Build history of the part. All positions in model axes, mm. A direction names the side the tool comes from. Give positions to 0.01 mm unless a question says otherwise; leave off trailing zeros. Loops run counter-clockwise (first coordinate to the right, second up) from the corner with the lowest first, then second, coordinate; pieces in that order, holes last. Notation, with made-up numbers: (17.25, 11.5) -> (40.25, 11.5) arc R25 cw to (40.25, 43.5) -> close; hole circle Ø11 at (85.25, -3.5). An arc over 180 degrees is marked (long way). One line per question, with ' | ' between items. Start each with the question number.
(1) Drill centre lines: L1, parallel to X at y = -5, z = 2.5; L2, parallel to Y at x = -34, z = 1; L3, parallel to Z at x = -31.5, y = 5 (3 decimals). Where is each one in solid material? Low to high. Write a range as from..to.
(2) Slice it at B-B, the plane z = 5.75. Write the cut outline in (x, y), then the cut area to 3 significant figures.
(3) Slice it at D-D, the plane y = 12. Write the cut outline in (x, z) (1 decimal).
(4) Slice it at C-C, the plane x = -11. Write the cut outline in (y, z) (1 decimal), then the cut area to 3 significant figures.
(5) 3-axis set-ups, long thin cutter, end or side, ignore diameter. For faces 1 (the face through (-21.9, 51.7, 1.588)), 2 (the face through (-33, 37.505, 2)), 3 (the face through (-14.31, 14.69, 4.94)): which of +Z, -Z, +X, -X, +Y, -Y reach the whole face in a straight line?
(6) Slice it at A-A, the plane x = 4.5. Write the cut outline in (y, z) (1 decimal), then the cut area to 3 significant figures.
(7) Flat gauge pins, fed straight in: pin 1 Ø6 at (x, y) = (-23.5, 43.5) entering from -Z; pin 2 Ø1.7 at (y, z) = (39, 2.5) entering from -X; pin 3 Ø1.7 at (x, z) = (-8, 2.5) entering from -Y; pin 4 Ø3.5 at (x, y) = (-21.5, 51) entering from +Z. Where does each tip first touch, or does it go through?
(8) Mould opens along X. For faces 4 (the face through (-22.97, 21.01, 4.94)), 5 (the face through (-14.46, 29.388, 3.421)), 6 (the face through (-7, -1.588, 2)), 7 (the face through (5.674, -5.551, 1.565)) say: pulls with the +X half, pulls with the -X half, needs draft (parallel to the pull), parting line crosses it, or undercut.
Autodesk Inventor part; units mm, degrees
ref_plane "YZ Plane" through (0, 0, 0) normal (1, 0, 0) x (0, 1, 0)
ref_plane "XZ Plane" through (0, 0, 0) normal (0, 1, 0) x (-1, 0, 0)
ref_plane "XY Plane" through (0, 0, 0) normal (0, 0, 1) x (1, 0, 0)
sketch "Sketch27" plane through (0, 0, 0) normal (0, 0, 1) x (1, 0, 0)
  line L0 (0, -7.9375) -> (-28.575, -7.9375)
  line L1 (-36.5125, 0) -> (-36.5125, 47.625)
  line L2 (-28.575, 55.5625) -> (0, 55.5625)
  line L3 (7.9375, 47.625) -> (7.9375, 0)
  circle A0 centre (-28.575, 47.625) radius 6.5484
  circle A1 centre (-28.575, 31.75) radius 6.5484
  circle A2 centre (-28.575, 15.875) radius 6.5484
  circle A3 centre (-28.575, 0) radius 6.5484
  circle A4 centre (-14.2875, 0) radius 6.5484
  circle A5 centre (-14.2875, 47.625) radius 6.5484
  circle A6 centre (0, 47.625) radius 6.5484
  circle A7 centre (0, 31.75) radius 6.5484
  circle A8 centre (0, 15.875) radius 6.5484
  circle A9 centre (0, 0) radius 6.5484
  arc A10 (-28.575, 55.5625) -> (-36.5125, 47.625) centre (-28.575, 47.625) ccw
  arc A11 (7.9375, 47.625) -> (0, 55.5625) centre (0, 47.625) ccw
  arc A12 (-36.5125, 0) -> (-28.575, -7.9375) centre (-28.575, 0) ccw
  arc A13 (0, -7.9375) -> (7.9375, 0) centre (0, 0) ccw
  circle A14 centre (-33.3375, 39.6875) radius 1.3891
  circle A15 centre (-33.3375, 23.8125) radius 1.3891
  circle A16 centre (-33.3375, 7.9375) radius 1.3891
  circle A17 centre (4.7625, 39.6875) radius 1.3891
  circle A18 centre (4.7625, 23.8125) radius 1.3891
  circle A19 centre (4.7625, 7.9375) radius 1.3891
  circle A20 centre (-21.4312, 53.1812) radius 1.3891
  circle A21 centre (-7.1437, 53.1812) radius 1.3891
  circle A22 centre (-21.4312, -5.5562) radius 1.3891
  circle A23 centre (-7.1437, -5.5562) radius 1.3891
  dimension "d126" = 13.0969
  dimension "d127" = 13.0969
  dimension "d128" = 13.0969
  dimension "d129" = 13.0969
  dimension "d130" = 13.0969
  dimension "d131" = 13.0969
  dimension "d132" = 13.0969
  dimension "d133" = 13.0969
  dimension "d134" = 13.0969
  dimension "d135" = 13.0969
  dimension "d136" = 7.9375
  dimension "d137" = 14.2875
  dimension "d138" = 14.2875
  dimension "d139" = 7.9375
  dimension "d140" = 7.9375
  dimension "d141" = 15.875
  dimension "d142" = 15.875
  dimension "d145" = 44.45
  dimension "d146" = 63.5
  dimension "d149" = 2.7781
  dimension "d150" = 2.7781
  dimension "d151" = 2.7781
  dimension "d152" = 2.7781
  dimension "d153" = 2.7781
  dimension "d154" = 2.7781
  dimension "d155" = 3.175
  dimension "d156" = 3.175
  dimension "d157" = 15.875
  dimension "d158" = 15.875
  dimension "d159" = 15.875
  dimension "d162" = 2.7781
  dimension "d163" = 2.7781
  dimension "d164" = 2.7781
  dimension "d165" = 2.7781
  dimension "d166" = 2.3813
  dimension "d169" = 2.3813
  dimension "d170" = 7.1437
  dimension "d171" = 7.1437
extrude "Extrusion25" add sketch "Sketch27" along normal blind 3.175 contours L0 A12 L1 A10 L2 A11 L3 A13 | A0 | A1 | A2 | A3 | A4 | A5 | A6 | A7 | A8 | A9
sketch "Sketch38" plane through (0, 0, 3.175) normal (0, 0, 1) x (1, 0, 0)
  circle A0 centre (-14.2875, 23.8125) radius 9.525
  arc A1 (-15.4885, 33.2615) -> (-18.8698, 32.1628) centre (-16.6896, 31.2053) ccw
  arc A2 (-15.4885, 33.2615) -> (-13.0865, 33.2615) centre (-14.2875, 35.3177) ccw
  line L0 (7.9375, 0) -> (7.9375, 47.625)
  line L1 (0, 55.5625) -> (-28.575, 55.5625)
  arc A3 (-9.7052, 32.1628) -> (-13.0865, 33.2615) centre (-11.8854, 31.2053) ccw
  arc A4 (-9.7052, 32.1628) -> (-7.7619, 30.7509) centre (-7.5249, 33.1204) ccw
  arc A5 (-5.6721, 27.8746) -> (-7.7619, 30.7509) centre (-7.9988, 28.3815) ccw
  arc A6 (-5.6721, 27.8746) -> (-4.9299, 25.5901) centre (-3.3454, 27.3678) ccw
  arc A7 (-4.9299, 22.0349) -> (-4.9299, 25.5901) centre (-6.5143, 23.8125) ccw
  arc A8 (-4.9299, 22.0349) -> (-5.6721, 19.7504) centre (-3.3454, 20.2572) ccw
  arc A9 (-7.7619, 16.8741) -> (-5.6721, 19.7504) centre (-7.9988, 19.2435) ccw
  arc A10 (-7.7619, 16.8741) -> (-9.7052, 15.4622) centre (-7.5249, 14.5046) ccw
  arc A11 (-13.0865, 14.3635) -> (-9.7052, 15.4622) centre (-11.8854, 16.4197) ccw
  arc A12 (-13.0865, 14.3635) -> (-15.4885, 14.3635) centre (-14.2875, 12.3073) ccw
  arc A13 (-18.8698, 15.4622) -> (-15.4885, 14.3635) centre (-16.6896, 16.4197) ccw
  arc A14 (-18.8698, 15.4622) -> (-20.8131, 16.8741) centre (-21.0501, 14.5046) ccw
  arc A15 (-22.9029, 19.7504) -> (-20.8131, 16.8741) centre (-20.5762, 19.2435) ccw
  arc A16 (-22.9029, 19.7504) -> (-23.6451, 22.0349) centre (-25.2296, 20.2572) ccw
  arc A17 (-20.8131, 30.7509) -> (-18.8698, 32.1628) centre (-21.0501, 33.1204) ccw
  arc A18 (-23.6451, 25.5901) -> (-23.6451, 22.0349) centre (-22.0607, 23.8125) ccw
  arc A19 (-23.6451, 25.5901) -> (-22.9029, 27.8746) centre (-25.2296, 27.3678) ccw
  arc A20 (-20.8131, 30.7509) -> (-22.9029, 27.8746) centre (-20.5762, 28.3815) ccw
  point P0 (0, 0)
  dimension "d265" = 19.05
  dimension "d266" = 22.225
  dimension "d267" = 31.75
  dimension "d268" = 2.3813
extrude "Extrusion29" add sketch "Sketch38" along normal blind 3.5719 contours A0 A8 A10 A12 A14 A16 A19 A17 A2 A4 A6 | A0 A7 | A0 A5 | A9 A0 | A0 A3 | A11 A0 | A0 A1 | A13 A0 | A0 A20 | A15 A0 | A0 A18
sketch "Sketch39" plane through (0, 0, 3.175) normal (0, 0, 1) x (1, 0, 0)
  line L0 (7.9375, 10.1203) -> (1.5875, 10.1203)
  line L1 (1.5875, 10.1203) -> (1.5875, 5.7547)
  line L2 (1.5875, 5.7547) -> (7.9375, 5.7547)
  line L3 (7.9375, 5.7547) -> (7.9375, 10.1203)
  line L4 (7.9375, 0) -> (7.9375, 47.625)
  circle A0 centre (4.7625, 7.9375) radius 1.3891
  line L5 (7.9375, 25.9953) -> (1.5875, 25.9953)
  line L6 (1.5875, 25.9953) -> (1.5875, 21.6297)
  line L7 (1.5875, 21.6297) -> (7.9375, 21.6297)
  line L8 (7.9375, 21.6297) -> (7.9375, 25.9953)
  line L9 (7.9375, 41.8703) -> (1.5875, 41.8703)
  line L10 (1.5875, 41.8703) -> (1.5875, 37.5047)
  line L11 (1.5875, 37.5047) -> (7.9375, 37.5047)
  line L12 (7.9375, 37.5047) -> (7.9375, 41.8703)
  line L13 (0, 55.5625) -> (-28.575, 55.5625)
  line L14 (-9.3266, 55.5625) -> (-4.9609, 55.5625)
  line L15 (-4.9609, 55.5625) -> (-4.9609, 49.2125)
  line L16 (-4.9609, 49.2125) -> (-9.3266, 49.2125)
  line L17 (-9.3266, 49.2125) -> (-9.3266, 55.5625)
  line L18 (-19.2484, 55.5625) -> (-23.6141, 55.5625)
  line L19 (-23.6141, 55.5625) -> (-23.6141, 49.2125)
  line L20 (-23.6141, 49.2125) -> (-19.2484, 49.2125)
  line L21 (-19.2484, 49.2125) -> (-19.2484, 55.5625)
  line L22 (-36.5125, 41.8703) -> (-30.1625, 41.8703)
  line L23 (-30.1625, 41.8703) -> (-30.1625, 37.5047)
  line L24 (-30.1625, 37.5047) -> (-36.5125, 37.5047)
  line L25 (-36.5125, 37.5047) -> (-36.5125, 41.8703)
  line L26 (-36.5125, 25.9953) -> (-30.1625, 25.9953)
  line L27 (-30.1625, 25.9953) -> (-30.1625, 21.6297)
  line L28 (-30.1625, 21.6297) -> (-36.5125, 21.6297)
  line L29 (-36.5125, 21.6297) -> (-36.5125, 25.9953)
  line L30 (-36.5125, 10.1203) -> (-30.1625, 10.1203)
  line L31 (-30.1625, 10.1203) -> (-30.1625, 5.7547)
  line L32 (-30.1625, 5.7547) -> (-36.5125, 5.7547)
  line L33 (-36.5125, 5.7547) -> (-36.5125, 10.1203)
  line L34 (0, -7.9375) -> (-28.575, -7.9375)
  line L35 (-23.6141, -7.9375) -> (-19.2484, -7.9375)
  line L36 (-19.2484, -7.9375) -> (-19.2484, -1.5875)
  line L37 (-19.2484, -1.5875) -> (-23.6141, -1.5875)
  line L38 (-23.6141, -1.5875) -> (-23.6141, -7.9375)
  line L39 (-9.3266, -7.9375) -> (-4.9609, -7.9375)
  line L40 (-4.9609, -7.9375) -> (-4.9609, -1.5875)
  line L41 (-4.9609, -1.5875) -> (-9.3266, -1.5875)
  line L42 (-9.3266, -1.5875) -> (-9.3266, -7.9375)
  line L43 (-36.5125, 47.625) -> (-36.5125, 0)
  circle A1 centre (4.7625, 23.8125) radius 1.3891
  circle A2 centre (4.7625, 39.6875) radius 1.3891
  circle A3 centre (-7.1437, 53.1812) radius 1.3891
  circle A4 centre (-21.4312, 53.1812) radius 1.3891
  point P0 (0, 0)
  dimension "d273" = 4.3656
  dimension "d274" = 6.35
  dimension "d275" = 2.1828
  dimension "d276" = 2.1828
  dimension "d277" = 2.1828
  dimension "d278" = 2.1828
  dimension "d279" = 2.1828
extrude "Extrusion30" cut sketch "Sketch39" against normal blind 1.5875
sketch "Sketch41" plane through (0, 0, 6.7469) normal (0, 0, 1) x (1, 0, 0)
  circle A0 centre (-14.2875, 30.1625) radius 0.7937
  circle A1 centre (-14.2875, 17.4625) radius 0.7937
  circle A2 centre (-7.9375, 23.8125) radius 0.7937
  circle A3 centre (-20.6375, 23.8125) radius 0.7937
  line L0 (-9.3266, 55.5625) -> (-19.2484, 55.5625)
  line L1 (7.9375, 25.9953) -> (7.9375, 37.5047)
  point P0 (0, 0)
  dimension "d287" = 1.5875
  dimension "d288" = 1.5875
  dimension "d289" = 1.5875
  dimension "d290" = 1.5875
  dimension "d291" = 12.7
  dimension "d292" = 12.7
  dimension "d293" = 6.35
  dimension "d294" = 6.35
  dimension "d295" = 25.4
  dimension "d296" = 15.875
extrude "Extrusion32" cut sketch "Sketch41" against normal through all
equation "\"d127\" = d126"
equation "\"d128\" = d126"
equation "\"d129\" = d126"
equation "\"d130\" = d126"
equation "\"d131\" = d126"
equation "\"d132\" = d126"
equation "\"d133\" = d126"
equation "\"d134\" = d126"
equation "\"d135\" = d126"
equation "\"d138\" = d137"
equation "\"d139\" = d136"
equation "\"d140\" = d136"
equation "\"d142\" = d141"
equation "\"d150\" = d149"
equation "\"d151\" = d149"
equation "\"d152\" = d149"
equation "\"d153\" = d149"
equation "\"d154\" = d149"
equation "\"d158\" = d157"
equation "\"d159\" = d157"
equation "\"d162\" = d149"
equation "\"d163\" = d149"
equation "\"d164\" = d149"
equation "\"d165\" = d149"
equation "\"d170\" = 0.5 * d137"
equation "\"d171\" = d170"
properties part number "magnetic1-1"
Final values:
1) L1: -34.74..-23.61, -19.25..-9.33, -4.96..6.16 | L2: -5.79..6.72, 9.16..22.59, 25.03..38.47, 40.91..53.42 | L3: 0..3.175
2) outline: (-23.65, 22.03) arc R2.38 cw to (-22.9, 19.75) arc R2.38 ccw to (-20.81, 16.87) arc R2.38 cw to (-18.87, 15.46) arc R2.38 ccw to (-15.49, 14.36) arc R2.38 cw to (-13.09, 14.36) arc R2.38 ccw to (-9.71, 15.46) arc R2.38 cw to (-7.76, 16.87) arc R2.38 ccw to (-5.67, 19.75) arc R2.38 cw to (-4.93, 22.03) arc R2.38 ccw to (-4.93, 25.59) arc R2.38 cw to (-5.67, 27.87) arc R2.38 ccw to (-7.76, 30.75) arc R2.38 cw to (-9.71, 32.16) arc R2.38 ccw to (-13.09, 33.26) arc R2.38 cw to (-15.49, 33.26) arc R2.38 ccw to (-18.87, 32.16) arc R2.38 cw to (-20.81, 30.75) arc R2.38 ccw to (-22.9, 27.87) arc R2.38 cw to (-23.65, 25.59) arc R2.38 ccw to start; hole circle Ø1.59 at (-20.64, 23.81); hole circle Ø1.59 at (-14.29, 17.46); hole circle Ø1.59 at (-14.29, 30.16); hole circle Ø1.59 at (-7.94, 23.81) | area: 286 mm2
3) outline: (-36.5, 0) -> (7.9, 0) -> (7.9, 3.2) -> (-36.5, 3.2) -> close
4) outline: (-7.9, 0) -> (55.6, 0) -> (55.6, 3.2) -> (33.4, 3.2) -> (33.4, 6.7) -> (14.2, 6.7) -> (14.2, 3.2) -> (-7.9, 3.2) -> close | area: 270 mm2
5) face 1: +Z, +Y | face 2: +Z, -X | face 3: +Z, -Y
6) outline: (-6.5, 0) -> (6.6, 0) -> (6.6, 1.6) -> (5.8, 1.6) -> (5.8, 3.2) -> (-6.5, 3.2) -> close; (9.3, 0) -> (22.4, 0) -> (22.4, 1.6) -> (21.6, 1.6) -> (21.6, 3.2) -> (10.1, 3.2) -> (10.1, 1.6) -> (9.3, 1.6) -> close; (25.2, 0) -> (38.3, 0) -> (38.3, 1.6) -> (37.5, 1.6) -> (37.5, 3.2) -> (26, 3.2) -> (26, 1.6) -> (25.2, 1.6) -> close; (41.1, 0) -> (54.2, 0) -> (54.2, 3.2) -> (41.9, 3.2) -> (41.9, 1.6) -> (41.1, 1.6) -> close | area: 159 mm2
7) pin 1: z = 0 | pin 2: x = -30.16 | pin 3: y = -1.59 | pin 4: z = 1.59
8) face 4: pulls with the -X half | face 5: undercut | face 6: undercut | face 7: pulls with the +X half
